from build123d import *

# Parameters (mm, degrees)
SKETCH1_W           = 80
SKETCH1_H           = 60
BOSS_EXTRUDE3_DEPTH = 10
SKETCH2_R           = 5.5
CUT_EXTRUDE2_DEPTH  = 7
SKETCH3_R           = 2
CUT_EXTRUDE3_DEPTH  = 10
CUT_EXTRUDE4_DEPTH  = 8
SKETCH6_W           = 38
SKETCH6_H           = 2
CUT_EXTRUDE5_DEPTH  = 60
SKETCH7_R           = 3.3
CUT_EXTRUDE7_DEPTH  = 13


with BuildPart() as part:
    # Sketch1 → Boss-Extrude3 (new body)
    with BuildSketch(Plane(origin=(0, 0, 0), x_dir=(1, 0, 0), z_dir=(0, 1, 0))):
        with Locations((-30.040251739, 6.462955974)):
            Rectangle(SKETCH1_W, SKETCH1_H)
    extrude(amount=-BOSS_EXTRUDE3_DEPTH)

    # Sketch2 → Cut-Extrude2 (cut)
    with BuildSketch(Plane(origin=(0, 0, 0), x_dir=(1, 0, 0), z_dir=(0, 1, 0))):
        with Locations(Location((-62.540251739, 6.462955974, 0), (0, 0, 270))):
            Circle(SKETCH2_R)
        with Locations(Location((2.459748261, 6.462955974, 0), (0, 0, 270))):
            Circle(SKETCH2_R)
    extrude(amount=-CUT_EXTRUDE2_DEPTH, mode=Mode.SUBTRACT)

    # Sketch3 → Cut-Extrude3 (cut)
    with BuildSketch(Plane(origin=(0, 0, 0), x_dir=(1, 0, 0), z_dir=(0, 1, 0))):
        with Locations(Location((-62.540251739, 18.962955974, 0), (0, 0, 270))):
            Circle(SKETCH3_R)
        with Locations(Location((2.459748261, 18.962955974, 0), (0, 0, 270))):
            Circle(SKETCH3_R)
    extrude(amount=-CUT_EXTRUDE3_DEPTH, mode=Mode.SUBTRACT)

    # Sketch4 → Cut-Extrude4 (cut)
    with BuildSketch(Plane(origin=(0, 0, 0), x_dir=(1, 0, 0), z_dir=(0, 1, 0))):
        with BuildLine():
            Line((-43.040251739, 16.662955974), (-17.040251739, 16.662955974))
            ThreePointArc((-17.040251739, 16.662955974), (-15.48461682, 16.018590892), (-14.840251739, 14.462955974))
            Line((-14.840251739, 14.462955974), (-14.840251739, -1.537044026))
            ThreePointArc((-14.840251739, -1.537044026), (-15.48461682, -3.092678945), (-17.040251739, -3.737044026))
            Line((-17.040251739, -3.737044026), (-43.040251739, -3.737044026))
            ThreePointArc((-43.040251739, -3.737044026), (-44.595886658, -3.092678945), (-45.240251739, -1.537044026))
            Line((-45.240251739, -1.537044026), (-45.240251739, 14.462955974))
            ThreePointArc((-45.240251739, 14.462955974), (-44.595886658, 16.018590892), (-43.040251739, 16.662955974))
        make_face()
    extrude(amount=-CUT_EXTRUDE4_DEPTH, mode=Mode.SUBTRACT)

    # Sketch6 → Cut-Extrude5 (cut)
    with BuildSketch(Plane.XY.offset(23.537044026)):
        with Locations((-30.040251739, -9)):
            Rectangle(SKETCH6_W, SKETCH6_H)
    extrude(amount=-CUT_EXTRUDE5_DEPTH, mode=Mode.SUBTRACT)

    # Sketch7 → Cut-Extrude7 (cut)
    with BuildSketch(Plane(origin=(0, 0, 0), x_dir=(1, 0, 0), z_dir=(0, 1, 0))):
        with Locations(Location((-62.540251739, 6.462955974, 0), (0, 0, 270))):
            Circle(SKETCH7_R)
        with Locations(Location((2.459748261, 6.462955974, 0), (0, 0, 270))):
            Circle(SKETCH7_R)
    extrude(amount=-CUT_EXTRUDE7_DEPTH, mode=Mode.SUBTRACT)


solid = part.part
Geometry: final body of the model. Coordinates: model frame, mm. A direction names the side the tool comes from. Round coordinates to 2 decimals unless told otherwise and drop trailing zeros. Loops run counter-clockwise (first coordinate to the right, second up) from the corner with the lowest first, then second, coordinate; pieces in that order, holes last. Notation, with made-up numbers: (68.25, 81) - (99.25, 81) arc R19 ccw to (99.25, 114) - close; hole circle Ø6 at (58, 50.25). An arc over 180 degrees is marked (long way). Write each question's results on one line, items separated by ' | '. Start each with the question number.
1) Mould query, pull axis X, two halves, no side actions, for faces 1 (the face through (-0.887, -3.451, -10.828)), 2 (the face through (-3, -10, -7)), 3 (the face through (-70.04, -5, -6)). Classes: released by +X, released by -X, zero draft, split by the parting line, or undercut.
2) Cut plane B-B on x = -36. Return loops of the section in (y, z).
3) Line query: probe 1 along X at (y, z) = (-1.5, -11); probe 2 along Z at (x, y) = (-27, -6.5); probe 3 along X at (y, z) = (-4.75, -13.5). Output: solid intervals per line, ascending. Write a range as [from, to].
4) Cut plane A-A on y = -9. Return loops of the section in (x, z).
5) First-contact query: P1, Ø7.5, axis at x = 2.46, z = -6.46, coming from the +Y side; P2, Ø19, axis at x = -33, z = 7, coming from the -Y side. Flat tips, straight axial feed; report the tip coordinate or a pass-through.
6) Access query for faces 4 (the face through (-67.9, -3.5, -7.7)), 5 (the face through (-49.04, -9, -6)), 6 (the face through (-15.502, -3.944, -16.036)). Directions: +Z, -Z, +X, -X, +Y, -Y. A direction counts if a zero-diameter tool reaches every point of the face in a straight line with its end or side. Return the directions, or none.
7) Cut plane D-D on z = -18.5. Return loops of the section in (x, y), then the cut area to 3 significant figures.
8) Cut plane C-C on z = -8.5. Return loops of the section in (x, y).
Verdict:
1) face 1: undercut | face 2: zero draft | face 3: released by -X
2) outline: (-8, -36.46) - (0, -36.46) - (0, -16.66) - (-8, -16.66) - close; (-8, 3.74) - (0, 3.74) - (0, 23.54) - (-8, 23.54) - close
3) probe 1: x = [-70.04, -65.65], [-59.43, -45.24], [-14.84, -0.65], [5.57, 9.96] | probe 2: z = [-36.46, -16.66], [3.74, 23.54] | probe 3: x = [-70.04, -45.24], [-14.84, 9.96]
4) outline: (-70.04, -36.46) - (-49.04, -36.46) - (-49.04, 23.54) - (-70.04, 23.54) - close; (-11.04, -36.46) - (9.96, -36.46) - (9.96, 23.54) - (-11.04, 23.54) - close; hole circle Ø6.6 at (-62.54, -6.46); hole circle Ø4 at (-62.54, -18.96); hole circle Ø6.6 at (2.46, -6.46); hole circle Ø4 at (2.46, -18.96)
5) P1: stops at y = -7 | P2: stops at y = -8
6) face 4: +Y | face 5: +Z, -Z, -Y | face 6: +Y, -Y
7) outline: (-70.04, -10) - (-64.49, -10) - (-64.49, 0) - (-70.04, 0) - close; (-60.59, -10) - (-49.04, -10) - (-49.04, -8) - (-11.04, -8) - (-11.04, -10) - (0.51, -10) - (0.51, 0) - (-60.59, 0) - close; (4.41, -10) - (9.96, -10) - (9.96, 0) - (4.41, 0) - close | area: 646 mm2
8) outline: (-70.04, -10) - (-65.14, -10) - (-65.14, -7) - (-67.65, -7) - (-67.65, 0) - (-70.04, 0) - close; (-59.94, -10) - (-49.04, -10) - (-49.04, -8) - (-45.24, -8) - (-45.24, 0) - (-57.43, 0) - (-57.43, -7) - (-59.94, -7) - close; (-14.84, -8) - (-11.04, -8) - (-11.04, -10) - (-0.14, -10) - (-0.14, -7) - (-2.65, -7) - (-2.65, 0) - (-14.84, 0) - close; (5.06, -10) - (9.96, -10) - (9.96, 0) - (7.57, 0) - (7.57, -7) - (5.06, -7) - close
